Part model, mm, in its own coordinate system. Coordinates: 2 decimals unless noted, no trailing zeros. Loops run counter-clockwise (first coordinate to the right, second up) from the corner with the lowest first, then second, coordinate; pieces in that order, holes last. Notation, with made-up numbers: M 81,-35.75 L 97,-35.75 A10 ccw 97,-27.75 Z; hole C 80.5,71 d7. An arc over 180 degrees is marked long. Answer as CSV lines item,"result". Start each with the question number.
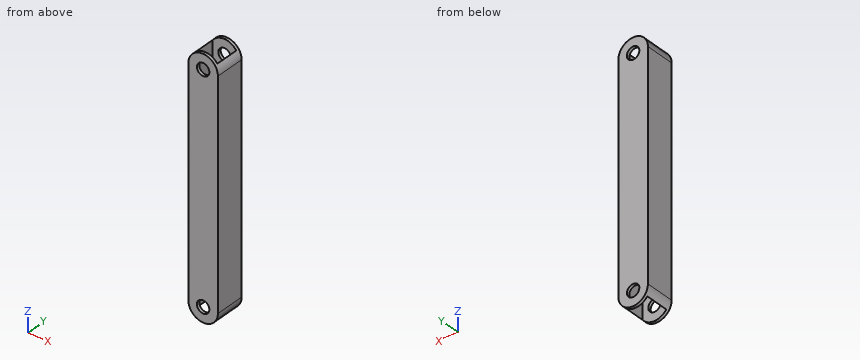
from build123d import *

# Parameters (mm, degrees)
SKETCH_1_W          = 10
SKETCH_1_H          = 10
SKETCH_1_W_2        = 8
SKETCH_1_H_2        = 8
EXTRUDE_1_DEPTH     = 85.374067158
SKETCH_2_R          = 2.1
CUT_EXTRUDE_1_DEPTH = 40
FILLET_1_R          = 5


with BuildPart() as part:
    # ｽｹｯﾁ1 → ﾎﾞｽ - 押し出し1 (new body)
    with BuildSketch(Plane.XY):
        Rectangle(SKETCH_1_W, SKETCH_1_H)
        Rectangle(SKETCH_1_W_2, SKETCH_1_H_2, mode=Mode.SUBTRACT)
    extrude(amount=EXTRUDE_1_DEPTH)

    # ｽｹｯﾁ2 → ｶｯﾄ - 押し出し1 (cut)
    with BuildSketch(Plane(origin=(0, 5, 0), x_dir=(1, 0, 0), z_dir=(0, 1, 0))):
        with Locations(Location((0, -5, 0), (0, 0, 270))):
            Circle(SKETCH_2_R)
        with Locations(Location((0, -80.374067158, 0), (0, 0, 270))):
            Circle(SKETCH_2_R)
    extrude(amount=-CUT_EXTRUDE_1_DEPTH, mode=Mode.SUBTRACT)

    # ﾌｨﾚｯﾄ1
    # the kernel refuses this fillet: 5 mm, written as the material it takes off along each edge
    with BuildSketch(Plane(origin=(5, 17.5, 85.374067158), x_dir=(-1, 0, 0), z_dir=(0, -1, 0)), Plane(origin=(-5, -17.5, 0), x_dir=(0, 0, 1), z_dir=(0, 1, 0))) as fillet_1_piece_1:
        with BuildLine():
            CenterArc((FILLET_1_R, FILLET_1_R), FILLET_1_R, 180, 90)
            Line((0, FILLET_1_R), (0, 0))
            Line((0, 0), (FILLET_1_R, 0))
        make_face()
    extrude(amount=35, mode=Mode.SUBTRACT)
    with BuildSketch(Plane(origin=(-5, -17.5, 85.374067158), x_dir=(0, 0, -1), z_dir=(0, 1, 0)), Plane(origin=(5, 17.5, 0), x_dir=(-1, 0, 0), z_dir=(0, -1, 0))) as fillet_1_piece_2:
        with BuildLine():
            CenterArc((FILLET_1_R, -FILLET_1_R), FILLET_1_R, 90, 90)
            Line((0, -FILLET_1_R), (0, 0))
            Line((0, 0), (FILLET_1_R, 0))
        make_face()
    extrude(amount=35, mode=Mode.SUBTRACT)


solid = part.part
Q1. Slice it at B-B, the plane y = -3.25. Write the cut outline in (x, z), and give its area (3 significant figures).
Q2. Wall check: L1, parallel to X at y = -3.25, z = 29.5; L2, parallel to X at y = 4.5, z = 5. Give the ranges that are in metal, low to high.
Q3. Slice it at A-A, the plane z = 65. Write the cut outline in (x, y).
Q4. Slice it at C-C, the plane z = 79.5. Write the cut outline in (x, y), and give its area (3 significant figures).
Solved:
1,outline,"M -5,5 A5 ccw -4,2 L -4,83.37 A5 ccw -5,80.37 Z; M 4,2 A5 ccw 5,5 L 5,80.37 A5 ccw 4,83.37 Z"
1,area,"159 mm2"
2,L1,"x = -5 to -4, 4 to 5"
2,L2,"x = -5 to -2.1, 2.1 to 5"
3,outline,"M -5,-5 L 5,-5 L 5,5 L -5,5 Z; hole M -4,-4 L 4,-4 L 4,4 L -4,4 Z"
4,outline,"M -5,-5 L -1.91,-5 L -1.91,-4 L -4,-4 L -4,4 L -1.91,4 L -1.91,5 L -5,5 Z; M 1.91,-5 L 5,-5 L 5,5 L 1.91,5 L 1.91,4 L 4,4 L 4,-4 L 1.91,-4 Z"
4,area,"28.4 mm2"
